The figure shows three views and two pictorial views of one solid part (mm, origin at its lowest corner). Answer the questions. A direction names the side the tool comes from. Give positions to 0.01 mm unless a question says otherwise; leave off trailing zeros. Loops run counter-clockwise (first coordinate to the right, second up) from the corner with the lowest first, then second, coordinate; pieces in that order, holes last. Notation, with made-up numbers: (19, -3) - (64, -3) arc R29 cw to (64, 24) - close; hole circle Ø6 at (10, -23.75). An arc over 180 degrees is marked (long way). Use a Markdown table: item, result. Add a question column.
Item 1: For a pull along X with two mould halves and no side action, classify the marked faces 3, 4, 5 and 6 as +X half, -X half, draft (parallel to the pull), parting line (faces both ways), or undercut.
Item 2: Consider probe 1 along Y at (x, z) = (2.8, 50); probe 2 along X at (y, z) = (165.5, 90.5); probe 3 along Y at (x, z) = (31.5, 40). Determine where each line is inside the solid, lowest interval first. Write a range as [from, to].
Item 3: A cutting plane is placed at C-C (y = 165). Determine the outline of the cut face in (x, z), plus the area to 3 significant figures.
Item 4: Which of the six approach directions +Z, -Z, +X, -X, +Y, -Y give full straight-line access (tool end or side, diameter ignored) to the marked faces 1 and 2?
Item 5: This flat-tipped pin is pushed along its axis until it touches: P1, Ø12, axis at x = 175, z = 47, coming from the +Y side. Where does it stop, or does it pass through?
Item 6: A cutting plane is placed at B-B (z = 50). Determine the outline of the cut face in (x, y).
Item 7: A cutting plane is placed at D-D (z = 29.5). Determine the outline of the cut face in (x, y).
Item 8: A cutting plane is placed at A-A (y = 30). Determine the outline of the cut face in (x, z).
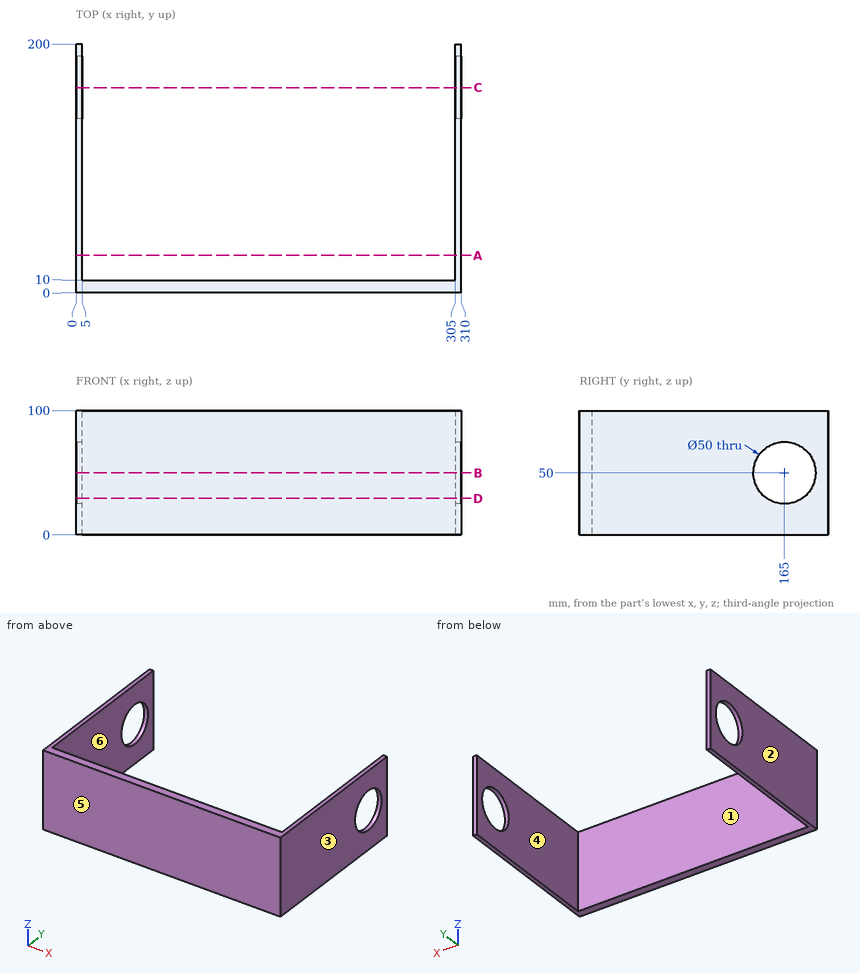
Geometry says:
| question | item | result |
|---|---|---|
| 1 | face 3 | +X half |
| 1 | face 4 | undercut |
| 1 | face 5 | draft |
| 1 | face 6 | undercut |
| 2 | probe 1 | [0, 140], [190, 200] |
| 2 | probe 2 | [0, 5], [305, 310] |
| 2 | probe 3 | [0, 10] |
| 3 | outline | (0, 0) - (5, 0) - (5, 25) - (0, 25) - close; (0, 75) - (5, 75) - (5, 100) - (0, 100) - close; (305, 0) - (310, 0) - (310, 25) - (305, 25) - close; (305, 75) - (310, 75) - (310, 100) - (305, 100) - close |
| 3 | area | 500 mm² |
| 4 | face 1 | +Z, -Z, +Y |
| 4 | face 2 | +Z, -Z, -X, +Y, -Y |
| 5 | P1 | y = 10 |
| 6 | outline | (0, 0) - (310, 0) - (310, 140) - (305, 140) - (305, 10) - (5, 10) - (5, 140) - (0, 140) - close; (0, 190) - (5, 190) - (5, 200) - (0, 200) - close; (305, 190) - (310, 190) - (310, 200) - (305, 200) - close |
| 7 | outline | (0, 0) - (310, 0) - (310, 150.69) - (305, 150.69) - (305, 10) - (5, 10) - (5, 150.69) - (0, 150.69) - close; (0, 179.31) - (5, 179.31) - (5, 200) - (0, 200) - close; (305, 179.31) - (310, 179.31) - (310, 200) - (305, 200) - close |
| 8 | outline | (0, 0) - (5, 0) - (5, 100) - (0, 100) - close; (305, 0) - (310, 0) - (310, 100) - (305, 100) - close |
